Design review of the part built by this model. Coordinates are the model's own, in mm. Face numbers are marked on the shaded views. A direction names the side the tool comes from. Give positions to 0.01 mm unless a question says otherwise; leave off trailing zeros. Loops run counter-clockwise (first coordinate to the right, second up) from the corner with the lowest first, then second, coordinate; pieces in that order, holes last. Notation, with made-up numbers: (82.5, 29.5) -> (140.5, 29.5) arc R18 ccw to (140.5, 52.5) -> close; hole circle Ø4 at (-3.5, 5.25). An arc over 180 degrees is marked (long way). Answer as CSV lines item,"result".
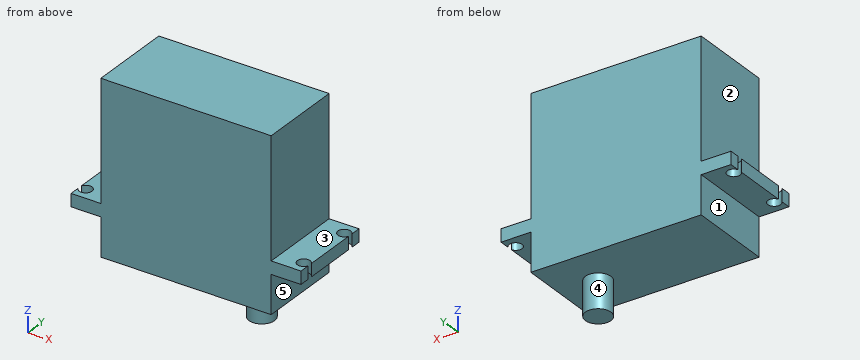
from build123d import *

# Parameters (mm, degrees)
ESQUISSE1_W             = 40
ESQUISSE1_H             = 20
BOSS_EXTRU_1_DEPTH      = 40
ESQUISSE3_W             = 3
ESQUISSE3_H             = 20
BOSS_EXTRU_2_DEPTH      = 7
ESQUISSE4_W             = 3
ESQUISSE4_H             = 20
BOSS_EXTRU_3_DEPTH      = 7
ESQUISSE5_R             = 1.5
ENL_V_MAT_EXTRU_3_DEPTH = 7
ESQUISSE6_R             = 3
BOSS_EXTRU_4_DEPTH      = 8


with BuildPart() as part:
    # Esquisse1 → Boss.-Extru.1 (new body)
    with BuildSketch(Plane.XY):
        with Locations((20, 10)):
            Rectangle(ESQUISSE1_W, ESQUISSE1_H)
    extrude(amount=BOSS_EXTRU_1_DEPTH)

    # Esquisse3 → Boss.-Extru.2 (add)
    with BuildSketch(Plane(origin=(40, 0, 0), x_dir=(0, 0, -1), z_dir=(1, 0, 0))):
        with Locations((-10.5, 10)):
            Rectangle(ESQUISSE3_W, ESQUISSE3_H)
    extrude(amount=BOSS_EXTRU_2_DEPTH)

    # Esquisse4 → Boss.-Extru.3 (add)
    with BuildSketch(Plane.ZY):
        with Locations((10.5, 10)):
            Rectangle(ESQUISSE4_W, ESQUISSE4_H)
    extrude(amount=BOSS_EXTRU_3_DEPTH)

    # Esquisse5 → Enlèv. mat.-Extru.3 (cut)
    with BuildSketch(Plane(origin=(0, 0, 9), x_dir=(-1, 0, 0), z_dir=(0, 0, -1))):
        with Locations((-45.6, 17)):
            Circle(ESQUISSE5_R)
        with Locations((-45.6, 3)):
            Circle(ESQUISSE5_R)
        with Locations((5.6, 17)):
            Circle(ESQUISSE5_R)
        with Locations((5.6, 3)):
            Circle(ESQUISSE5_R)
    extrude(amount=-ENL_V_MAT_EXTRU_3_DEPTH, mode=Mode.SUBTRACT)

    # Esquisse6 → Boss.-Extru.4 (add)
    with BuildSketch(Plane(origin=(0, 0, 0), x_dir=(-1, 0, 0), z_dir=(0, 0, -1))):
        with Locations((-31, 10)):
            Circle(ESQUISSE6_R)
    extrude(amount=BOSS_EXTRU_4_DEPTH)


solid = part.part
Q1. Clearance check with flat-ended pins moving along their axes: pin 1 Ø4 at (x, y) = (45.6, 17) entering from -Z; pin 2 Ø2 at (x, y) = (42.5, 5) entering from +Z; pin 3 Ø12 at (y, z) = (8.5, -2.5) entering from +X; pin 4 Ø1.8 at (x, y) = (-5.6, 3) entering from -Z. State where each tip first meets the part, or that it passes through.
Filled sheet:
pin 1,"stops at z = 9"
pin 2,"stops at z = 12"
pin 3,"stops at x = 40"
pin 4,"passes through"
Q2. We need section C-C, the plane x = 31. State the section outline as (y, z) points.
Filled sheet:
outline,"(0, 0) -> (7, 0) -> (7, -8) -> (13, -8) -> (13, 0) -> (20, 0) -> (20, 40) -> (0, 40) -> close"
Q3. We need section A-A, the plane x = -5.6. State the section outline as (y, z) points, and give its area (3 significant figures).
Filled sheet:
outline,"(0, 9) -> (1.5, 9) -> (1.5, 12) -> (0, 12) -> close; (4.5, 9) -> (15.5, 9) -> (15.5, 12) -> (4.5, 12) -> close; (18.5, 9) -> (20, 9) -> (20, 12) -> (18.5, 12) -> close"
area,"42.0 mm^2"
Q4. To check wall thickness, follow probe 1 along Y at (x, z) = (45.6, 11.25); probe 2 along Z at (x, y) = (23.5, 17); probe 3 along Z at (x, y) = (-1.5, 10). State the ranges of each line that lie inside material, in increasing order. Write a range as from..to.
Filled sheet:
probe 1,"y = 0..1.5, 4.5..15.5, 18.5..20"
probe 2,"z = 0..40"
probe 3,"z = 9..12"
Q5. We need section D-D, the plane z = -1. State the section outline as (x, y) points.
Filled sheet:
outline,"circle Ø6 at (31, 10)"
Q6. For the marked faces 1, 2, 3, 4 and 5, list the 3-axis set-ups (+Z, -Z, +X, -X, +Y, -Y) from which the entire face can be reached by the end or side of a thin tool; tool diameter is ignored.
Filled sheet:
face 1,"-Z, -X, +Y, -Y"
face 2,"+Z, -X, +Y, -Y"
face 3,"+Z, +X, +Y, -Y"
face 4,"-Z"
face 5,"-Z, +X, +Y, -Y"
Q7. We need section B-B, the plane y = 14.5. State the section outline as (x, z) points, and give its area (3 significant figures).
Filled sheet:
outline,"(-7, 9) -> (0, 9) -> (0, 0) -> (40, 0) -> (40, 9) -> (47, 9) -> (47, 12) -> (40, 12) -> (40, 40) -> (0, 40) -> (0, 12) -> (-7, 12) -> close"
area,"1,640 mm^2"
